Autodesk Inventor part; units mm, degrees
ref_plane "YZ Plane" through (0, 0, 0) normal (1, 0, 0) x (0, 1, 0)
ref_plane "XZ Plane" through (0, 0, 0) normal (0, 1, 0) x (-1, 0, 0)
ref_plane "XY Plane" through (0, 0, 0) normal (0, 0, 1) x (1, 0, 0)
sketch "Эскиз1" plane through (0, 0, 0) normal (0, 0, 1) x (1, 0, 0)
  line L0 (-30.5, 15) -> (30.5, 15)
  line L1 (30.5, 15) -> (30.5, -15)
  line L2 (30.5, -15) -> (-30.5, -15)
  line L3 (-30.5, -15) -> (-30.5, 15)
  line L4 (0, -24.15) -> (0, 24.15)
  line L5 (-45.5, 0) -> (45.5, 0)
  line L6 (-32.5, 17.25) -> (32.5, 17.25)
  line L7 (32.5, 17.25) -> (32.5, -17.25)
  line L8 (32.5, -17.25) -> (-32.5, -17.25)
  line L9 (-32.5, -17.25) -> (-32.5, 17.25)
  point P0 (0, 0)
  dimension "d0" = 61
  dimension "d1" = 30
  dimension "d2" = 34.5
  dimension "d3" = 65
extrude "Выдавливание1" add sketch "Эскиз1" along normal blind 3
extrude "Выдавливание2" add sketch "Эскиз1" against normal blind 80 contours L3 L5 L9 L6 L4 L0 | L4 L6 L7 L5 L1 L0 | L3 L2 L4 L8 L9 L5 | L5 L7 L8 L4 L2 L1
sketch "Эскиз2" plane through (0, 0, 3) normal (0, 0, 1) x (1, 0, 0)
  circle A0 centre (-10, 0) radius 5.6
  circle A1 centre (10, 0) radius 5.6
  line L0 (0, -24.15) -> (0, 24.15)
  point P0 (0, 0)
  dimension "d8" = 20
  dimension "d9" = 11.2
  dimension "d10" = 11.2
extrude "Выдавливание3" cut sketch "Эскиз2" against normal blind 80
sketch "Эскиз3" plane through (0, 0, -80) normal (0, 0, -1) x (-1, 0, 0)
  line L0 (30.5, -15) -> (-30.5, -15)
  circle A0 centre (-10, 0) radius 5.6
  circle A1 centre (10, 0) radius 5.6
  line L1 (-30.5, -15) -> (30.5, -15)
  line L2 (30.5, -15) -> (30.5, 15)
  line L3 (30.5, 15) -> (-30.5, 15)
  line L4 (-30.5, 15) -> (-30.5, -15)
  line L5 (32.5, -17.25) -> (-32.5, -17.25)
  line L6 (-35.7, -14.05) -> (-35.7, 14.05)
  line L7 (-32.5, 17.25) -> (32.5, 17.25)
  line L8 (35.7, 14.05) -> (35.7, -14.05)
  line L9 (0, -28.8249) -> (0, 30.0984)
  line L10 (57.8663, 0) -> (-57.8663, 0)
  line L11 (32.5, -17.25) -> (32.5, 17.25)
  line L12 (-32.5, 17.25) -> (-32.5, -17.25)
  arc A2 (32.5, -17.25) -> (35.7, -14.05) centre (32.5, -14.05) ccw
  arc A3 (35.7, 14.05) -> (32.5, 17.25) centre (32.5, 14.05) ccw
  arc A4 (-32.5, 17.25) -> (-35.7, 14.05) centre (-32.5, 14.05) ccw
  arc A5 (-35.7, -14.05) -> (-32.5, -17.25) centre (-32.5, -14.05) ccw
  point P0 (0, 0)
  point P1 (35.7, -17.25)
  point P2 (-30.5, -15)
  dimension "d13" = 3.2
  dimension "d14" = 3.2
  dimension "d15" = 3.2
extrude "Выдавливание4" add sketch "Эскиз3" along normal blind 2 contours L2 L10 L11 L5 L9 L0 | L9 L5 L12 L10 L4 L0 | L2 L3 L9 L7 L11 L10 | L11 A3 L8 L10 | L10 L8 A2 L11 | L10 L12 L7 L9 L3 L4 | A5 L6 L10 L12 | L10 L6 A4 L12
sketch "Эскиз4" plane through (0, 0, -82) normal (0, 0, -1) x (-1, 0, 0)
  line L0 (35.7, -14.05) -> (35.7, 14.05)
  arc A0 (35.7, -3.2879) -> (35.7, 3.2879) centre (34.5, 0) ccw
  line L1 (30.5, 15) -> (30.5, -15)
  arc A1 (35.7, -4.337) -> (35.7, 4.337) centre (34.5, 0) ccw
  line L2 (0, 0) -> (0, 3.9976)
  line L3 (-35.7, 14.05) -> (-35.7, -14.05)
  arc A2 (-35.7, 3.2879) -> (-35.7, -3.2879) centre (-34.5, 0) ccw
  arc A3 (-35.7, 4.337) -> (-35.7, -4.337) centre (-34.5, 0) ccw
  circle A4 centre (34.5, 0) radius 1.7
  circle A5 centre (-34.5, 0) radius 1.7
  point P0 (28.7, 0)
  point P1 (30.5, 0)
  point P2 (31, 0)
  point P3 (-35.7, -4.4956)
  point P4 (-35.7, 4.4956)
  dimension "d19" = 7
  dimension "d20" = 4
  dimension "d21" = 1
  dimension "d26" = 3.4
  dimension "d27" = 3.4
extrude "Выдавливание5" add sketch "Эскиз4" against normal blind 2 contours L0 A0 A1 | L0 A4 A0 | L0 A4 picked at (35.8557, 0.1108)
extrude "Выдавливание6" add sketch "Эскиз4" against normal blind 2 contours L3 A2 A3 | L3 A5 A2 | L3 A5 picked at (-35.7794, -0.3021)
extrude "Выдавливание7" cut sketch "Эскиз4" against normal blind 2 contours A4 L0 | L0 A4 | A5 L3 | L3 A5
fillet "Сопряжение1" radius 3 4 edges at (35.7, -4.337, -81) (35.7, 4.337, -81) (-35.7, -4.337, -81) (-35.7, 4.337, -81)
sketch "Эскиз5" plane through (0, 0, 3) normal (0, 0, 1) x (1, 0, 0)
  line L0 (32.5, 17.25) -> (-32.5, 17.25)
  circle A0 centre (10, 0) radius 5.6
  circle A1 centre (-10, 0) radius 5.6
  line L1 (32.5, 17.25) -> (-32.5, 17.25)
  line L2 (-32.5, 17.25) -> (-32.5, -17.25)
  line L3 (-32.5, -17.25) -> (32.5, -17.25)
  line L4 (32.5, -17.25) -> (32.5, 17.25)
  point P0 (0, 0)
extrude "Выдавливание8" cut sketch "Эскиз5" against normal up to surface (3 mm away) contours L4 L3 L2 L0 | A0 | A1
sketch "Эскиз6" plane through (-32.5, -17.25, 0) normal (0, 0, 1) x (1, 0, 0)
  line L0 (63, 2.25) -> (2, 2.25)
  line L1 (2, 2.25) -> (2, 32.25)
  line L2 (2, 32.25) -> (63, 32.25)
  line L3 (63, 32.25) -> (63, 2.25)
  line L4 (0, 0) -> (0, 34.5)
  line L5 (65, 0) -> (0, 0)
  line L6 (65, 34.5) -> (65, 0)
  line L7 (0, 34.5) -> (65, 34.5)
  point P0 (32.5, 17.25)
extrude "Выдавливание9" cut sketch "Эскиз1" against normal blind 12 contours L3 L5 L9 L6 L4 L0 | L4 L6 L7 L5 L1 L0 | L3 L2 L4 L8 L9 L5 | L5 L7 L8 L4 L2 L1
sketch "Эскиз7" plane through (0, 0, -12) normal (0, 0, 1) x (1, 0, 0)
  line L0 (-32.5, 17.25) -> (32.5, 17.25)
  line L1 (-32.5, 17.25) -> (32.5, 17.25)
  line L2 (-32.5, -17.25) -> (-32.5, 17.25)
  line L3 (32.5, -17.25) -> (-32.5, -17.25)
  line L4 (32.5, 17.25) -> (32.5, -17.25)
  line L5 (30.5, -15) -> (30.5, 15)
  line L6 (-30.5, -15) -> (30.5, -15)
  line L7 (-30.5, 15) -> (-30.5, -15)
  line L8 (30.5, 15) -> (-30.5, 15)
  line L9 (-31.5, 16.25) -> (31.5, 16.25)
  line L10 (31.5, 16.25) -> (31.5, -16.25)
  line L11 (31.5, -16.25) -> (-31.5, -16.25)
  line L12 (-31.5, -16.25) -> (-31.5, 16.25)
  point P0 (0, 0)
  dimension "d35" = 1
  dimension "d36" = 1
  dimension "d37" = 1
  dimension "d38" = 1
extrude "Выдавливание10" cut sketch "Эскиз7" against normal up to surface (68 mm away) contours L0 L4 L3 L2
fillet "Сопряжение2" radius 2 8 edges at (31.5, 16.25, -46) (30.5, 15, -47) (30.5, -15, -47) (31.5, -16.25, -46) (-31.5, -16.25, -46) (-31.5, 16.25, -46) (-30.5, -15, -47) (-30.5, 15, -47)
sketch "Эскиз10" plane through (-29.5, 16.25, -12) normal (0, 1, 0) x (1, 0, 0)
  point P0 (29.5, -12)
properties part number "нижняя часть держателя аккумов"
Here's how the part is built. I have some questions about the finished solid (model axes, mm). A direction names the side the tool comes from. Give positions to 0.01 mm unless a question says otherwise; leave off trailing zeros. Write each loop counter-clockwise with the first axis right and the second up, starting at its lowest first coordinate (ties: lowest second). Pieces come first, ordered by that corner, then holes.
(1) Thinking about a two-plate mould opening in X: for faces 1 (the face through (-31.5, 0, -46)), 2 (the face through (0, -15, -47)), 3 (the face through (35.7, -10, -81)), which applies, pulls with the +X half, pulls with the -X half, needs draft (parallel to the pull), parting line crosses it, or undercut?
Output values:
face 1: pulls with the -X half
face 2: undercut
face 3: pulls with the +X half
(2) Imagine slicing it at B-B, the plane y = -7.5. Write out the boundary of the cut face in (x, z), and give its area (3 significant figures).
Output values:
outline: (-35.7, -82) - (-30.5, -82) - (-30.5, -12) - (-31.5, -12) - (-31.5, -80) - (-35.7, -80) - close; (30.5, -82) - (35.7, -82) - (35.7, -80) - (31.5, -80) - (31.5, -12) - (30.5, -12) - close
area: 157 mm2
(3) If I drill on L1, parallel to X at y = -7.5, z = -64; L2, parallel to Y at x = 28.5, z = -60.5; L3, parallel to Z at x = 35, y = -3, over which ranges is the centre line in solid material (lowest first)?
Output values:
L1: x = -31.5 to -30.5, 30.5 to 31.5
L2: y = -16.25 to -15, 15 to 16.25
L3: z = -82 to -80
(4) Imagine slicing it at C-C, the plane y = 0. Write out the boundary of the cut face in (x, z).
Output values:
outline: (-39, -82) - (-36.2, -82) - (-36.2, -80) - (-39, -80) - close; (-32.8, -82) - (-30.5, -82) - (-30.5, -12) - (-31.5, -12) - (-31.5, -80) - (-32.8, -80) - close; (30.5, -82) - (32.8, -82) - (32.8, -80) - (31.5, -80) - (31.5, -12) - (30.5, -12) - close; (36.2, -82) - (39, -82) - (39, -80) - (36.2, -80) - close
(5) Will these pins go through, and if not, where does the flat tip stop? pin 1 (0.6 mm diameter, centred on y = 8.5, z = -81, fed in from -X); pin 2 (8 mm diameter, centred on y = 1, z = -26, fed in from -X); pin 3 (0.6 mm diameter, centred on y = 11, z = -81.5, fed in from +X); pin 4 (12 mm diameter, centred on x = -25, y = -9, fed in from -Z).
Output values:
pin 1: stops at x = -35.7
pin 2: stops at x = -31.5
pin 3: stops at x = 35.7
pin 4: stops at z = -82
(6) Imagine slicing it at D-D, the plane z = -42. Write out the boundary of the cut face in (x, y), and give its area (4 significant figures).
Output values:
outline: (-31.5, -14.25) arc R2 ccw to (-29.5, -16.25) - (29.5, -16.25) arc R2 ccw to (31.5, -14.25) - (31.5, 14.25) arc R2 ccw to (29.5, 16.25) - (-29.5, 16.25) arc R2 ccw to (-31.5, 14.25) - close; hole (-30.5, -13) arc R2 ccw to (-28.5, -15) - (28.5, -15) arc R2 ccw to (30.5, -13) - (30.5, 13) arc R2 ccw to (28.5, 15) - (-28.5, 15) arc R2 ccw to (-30.5, 13) - close
area: 217.5 mm2
(7) Imagine slicing it at A-A, the plane x = -23. Write out the boundary of the cut face in (y, z).
Output values:
outline: (-17.25, -82) - (-15, -82) - (-15, -12) - (-16.25, -12) - (-16.25, -80) - (-17.25, -80) - close; (15, -82) - (17.25, -82) - (17.25, -80) - (16.25, -80) - (16.25, -12) - (15, -12) - close
(8) On a 3-axis mill with a long thin cutter (end or side, diameter ignored), from which of +Z, -Z, +X, -X, +Y, -Y can I reach the whole of each face in a straight line? I mean faces 4 (the face through (-30.93, 15.65, -46.48)), 5 (the face through (29.9, 14.43, -47.49)), 6 (the face through (-30.9, -15.68, -46.48)), 7 (the face through (30.9, 15.68, -46.48)), 8 (the face through (35.7, 10, -81)). Say none if no direction works.
Output values:
face 4: +Z, -X, +Y
face 5: +Z, -Z
face 6: +Z, -X, -Y
face 7: +Z, +X, +Y
face 8: +Z, -Z, +X, +Y
